Read the model definition and answer for the solid it produces. Units are mm, in the model's axes. A direction names the side the tool comes from. Give positions to 0.01 mm unless a question says otherwise; leave off trailing zeros. Order: outer loops, then holes, each group sorted by start corner. A loop starts at its lowest first (then second) coordinate and runs counter-clockwise, first axis right, second up. Notation, with made-up numbers: M 47.5,82 L 64.5,82 A21 cw 64.5,100 Z; hole C 77.25,-11.5 d9. An arc over 180 degrees is marked long. Write item = value, one per line. Start each with the question number.
Autodesk Inventor part; units mm, degrees
ref_plane "YZ Plane" through (0, 0, 0) normal (1, 0, 0) x (0, 1, 0)
ref_plane "XZ Plane" through (0, 0, 0) normal (0, 1, 0) x (-1, 0, 0)
ref_plane "XY Plane" through (0, 0, 0) normal (0, 0, 1) x (1, 0, 0)
sketch "Esboço1" plane through (0, 0, 0) normal (0, 0, 1) x (1, 0, 0)
  line L0 (0, 0) -> (9, 0)
  line L1 (9, 0) -> (9, 6.65)
  line L2 (9, 6.65) -> (0, 6.65)
  line L3 (0, 6.65) -> (0, 4.65)
  line L4 (0, 4.65) -> (2.5, 4.65)
  line L5 (2.5, 4.65) -> (2.5, 0)
  dimension "d0" = 9
  dimension "d1" = 6.65
  dimension "d2" = 2
  dimension "d3" = 2.5
revolve "Revolução1" add sketch "Esboço1" angle 360 about axis through (0, 0, 0) along (1, 0, 0)
sketch "Esboço2" plane through (9, 0, 0) normal (1, 0, 0) x (0, 0, -1)
  circle A0 centre (0, 0) radius 2
  dimension "d5" = 4
extrude "Extrusão1" add sketch "Esboço2" along normal blind 1.5
sketch "Esboço3" plane through (2.5, 0, 0) normal (-1, 0, 0) x (0, 0, 1)
  circle A0 centre (0, 0) radius 1.5
  dimension "d8" = 3
extrude "Extrusão2" cut sketch "Esboço3" against normal blind 4
sketch "Esboço4" plane through (0, 0, 0) normal (-1, 0, 0) x (0, 0, 1)
  point P0 (0, 0)
sketch "Esboço5" plane through (9, 0, 0) normal (1, 0, 0) x (0, 0, -1)
  point P0 (0, 0)
sketch "Esboço6" plane through (10.5, 0, 0) normal (1, 0, 0) x (0, 0, -1)
  circle A0 centre (0, 0) radius 2
  circle A1 centre (0, 0) radius 1
  dimension "d11" = 2
extrude "Extrusão3" cut sketch "Esboço6" against normal blind 1.06 contours A1
sketch "Esboço7" plane through (10.5, 0, 0) normal (1, 0, 0) x (0, 0, -1)
  circle A0 centre (0, 0) radius 2
extrude "Extrusão4" cut sketch "Esboço7" against normal blind 1.5
properties part number "roda sup"
1) For faces 5 (the face through (1.27, 2.5, 3.92)), 6 (the face through (9, 0, 0)), determine the directions among +Z, -Z, +X, -X, +Y, -Y from which every point of the face is accessible in a straight line to the end or side of a thin tool.
2) Find section C-C on x = 2. Determine the outline of the cut face in (y, z), plus the area to 3 significant figures.
3) For a pull along Z with two mould halves and no side action, classify faces 1 (the face through (0, -5, -1)), 2 (the face through (2.5, 2, 0)), 3 (the face through (4.44, 3.07, 5.9)), 4 (the face through (6.5, 0, 0)) as pulls with the +Z half, pulls with the -Z half, needs draft (parallel to the pull), parting line crosses it, or undercut.
4) Find section D-D on z = 0.5. Determine the outline of the cut face in (x, y).
5) Each of these flat-tipped pins is pushed along its axis until it touches: P1, Ø7.5, axis at y = -0.5, z = -2, coming from the -X side; P2, Ø3, axis at x = 4.5, z = 3, coming from the +Y side; P3, Ø4, axis at x = 6.5, z = 2.5, coming from the -Y side; P4, Ø2, axis at x = 2, z = -4, coming from the +Y side. Where does it stop, or does it pass through?
6) Find section B-B on z = -2.5. Determine the outline of the cut face in (x, y).
7) Find section A-A on y = 0. Determine the outline of the cut face in (x, z), plus the area to 4 significant figures.
8) Find the intervals of material crossed by probe 1 along Z at (x, y) = (1.1, 0); probe 2 along X at (y, z) = (-3.75, 2.5); probe 3 along Z at (x, y) = (0.75, -4), in increasing order. Write a range as [from, to].
Numbers:
q1.face_5 = -X
q1.face_6 = +Z, -Z, +X, +Y, -Y
q2.outline = C 0,0 d13.3; hole C 0,0 d9.3
q2.area = 71.0 mm2
q3.face_1 = needs draft
q3.face_2 = undercut
q3.face_3 = parting line crosses it
q3.face_4 = undercut
q4.outline = M 0,-6.63 L 9,-6.63 L 9,6.63 L 0,6.63 L 0,4.62 L 2.5,4.62 L 2.5,1.41 L 6.5,1.41 L 6.5,-1.41 L 2.5,-1.41 L 2.5,-4.62 L 0,-4.62 Z
q5.P1 = 0
q5.P2 = 6.48
q5.P3 = -6.63
q5.P4 = 5.93
q6.outline = M 0,-6.16 L 9,-6.16 L 9,6.16 L 0,6.16 L 0,3.92 L 2.5,3.92 L 2.5,-3.92 L 0,-3.92 Z
q7.outline = M 0,-6.65 L 9,-6.65 L 9,6.65 L 0,6.65 L 0,4.65 L 2.5,4.65 L 2.5,1.5 L 6.5,1.5 L 6.5,-1.5 L 2.5,-1.5 L 2.5,-4.65 L 0,-4.65 Z
q7.area = 84.45 mm2
q8.probe_1 = [-6.65, -4.65], [4.65, 6.65]
q8.probe_2 = [2.5, 9]
q8.probe_3 = [-5.31, -2.37], [2.37, 5.31]
